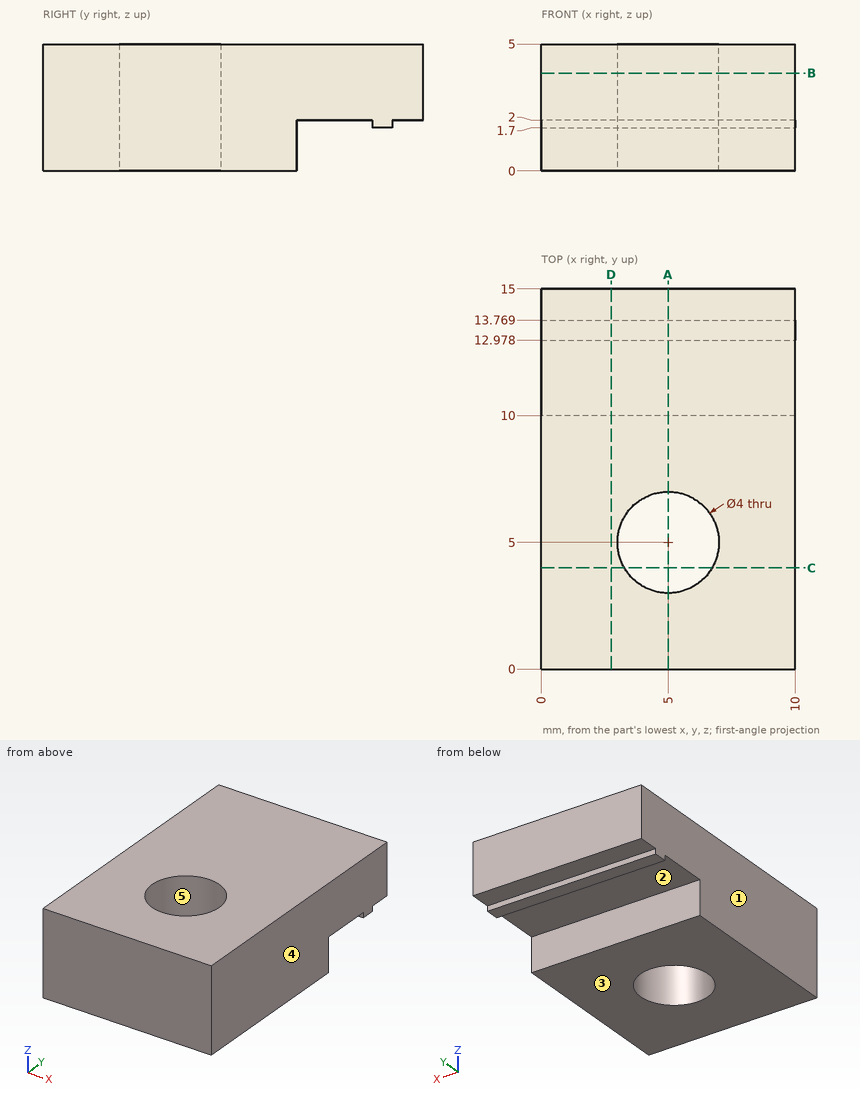
Design review of the part shown in the three views and the two pictorial views. Dimensions are in mm from the part's minimum x, y and z. A direction names the side the tool comes from. Coordinates: 2 decimals unless noted, no trailing zeros. Order: outer loops, then holes, each group sorted by start corner. A loop starts at its lowest first (then second) coordinate and runs counter-clockwise, first axis right, second up. Notation, with made-up numbers: (4.5, 10.5) - (62.5, 10.5) arc R12 ccw to (62.5, 25.5) - close; hole circle Ø11 at (16, 61). An arc over 180 degrees is marked (long way). Answer as CSV lines item,"result". Start each with the question number.
1) Draft analysis for pull direction X (two halves, no side actions). For the marked faces 3, 4 and 5, state which applies: +X half, -X half, draft (parallel to the pull), parting line (faces both ways), or undercut.
2) Machinability: for the marked faces 1 and 2, which of the approach directions +Z, -Z, +X, -X, +Y, -Y give a long, thin tool a straight path to every point of the face, cutting with its end or side? Answer none if there is none.
3) Insertion check: P1, Ø1.4, axis at x = 5.5, y = 14.5, coming from the -Z side. The pin has a flat end and moves straight along its axis. Give the tip position at first contact, or say it passes through.
4) To check wall thickness, follow line 1 along Y through (x, z) = (5, 1.8); line 2 along Y through (x, z) = (5, 3.5); line 3 along X through (y, z) = (5, 2.35). State the ranges of each line that lie inside material, in increasing order. Write a range as [from, to].
5) Add section C-C (y = 4). State the section outline as (x, z) points.
6) Add section D-D (x = 2.75). State the section outline as (y, z) points.
7) Add section B-B (z = 3.85). State the section outline as (x, y) points, then the cut area to 3 significant figures.
8) Add section A-A (x = 5). State the section outline as (y, z) points.
Result:
1,face 3,"draft"
1,face 4,"+X half"
1,face 5,"undercut"
2,face 1,"+Z, -Z, -X, +Y, -Y"
2,face 2,"-Z, +X, -X"
3,P1,"z = 2"
4,line 1,"[0, 3], [7, 10], [12.98, 13.77]"
4,line 2,"[0, 3], [7, 15]"
4,line 3,"[0, 3], [7, 10]"
5,outline,"(0, 0) - (3.27, 0) - (3.27, 5) - (0, 5) - close; (6.73, 0) - (10, 0) - (10, 5) - (6.73, 5) - close"
6,outline,"(0, 0) - (10, 0) - (10, 2) - (12.98, 2) - (12.98, 1.7) - (13.77, 1.7) - (13.77, 2) - (15, 2) - (15, 5) - (0, 5) - close"
7,outline,"(0, 0) - (10, 0) - (10, 15) - (0, 15) - close; hole circle Ø4 at (5, 5)"
7,area,"137 mm^2"
8,outline,"(0, 0) - (3, 0) - (3, 5) - (0, 5) - close; (7, 0) - (10, 0) - (10, 2) - (12.98, 2) - (12.98, 1.7) - (13.77, 1.7) - (13.77, 2) - (15, 2) - (15, 5) - (7, 5) - close"
